Here's how the part is built. I have some questions about the finished solid (model axes, mm). Face numbers are marked on the shaded views. A direction names the side the tool comes from. Coordinates: 2 decimals unless noted, no trailing zeros. Loops run counter-clockwise (first coordinate to the right, second up) from the corner with the lowest first, then second, coordinate; pieces in that order, holes last. Notation, with made-up numbers: (2, 13) -> (45, 13) arc R19 cw to (45, 35) -> close; hole circle Ø10 at (61.25, 12). An arc over 180 degrees is marked (long way). Answer as a JSON object with one key per item and string values. Group by question number.
1) I want a section at A-A (y = 0). Write out the boundary of the cut face in (x, z) (3 decimals), then the cut area to 3 significant figures.
2) I need wall thicknesses on probe 1 along Y at (x, z) = (0, 4.6) (3 decimals); probe 2 along Y at (x, z) = (0, 0.45); probe 3 along X at (y, z) = (0, 1). Which ranges of each line are inside material? Lowest first, please. Write a range as [from, to].
3) Which directions (+Z, -Z, +X, -X, +Y, -Y) give clear straight access to the entire face, cutting with the end or side of a thin tool? Please do the marked faces 1, 2 and 3.
4) I'm going to push flat-ended pins straight in: pin 1 (2 mm diameter, centred on x = -3.5, z = 5, fed in from +Y); pin 2 (2 mm diameter, centred on x = 2.5, z = 5, fed in from +Y); pin 3 (5.5 mm diameter, centred on x = 0, y = 0, fed in from +Z). Where does each tip first touch, or does it pass through?
5) I want a section at C-C (z = 1.3). Write out the boundary of the cut face in (x, y).
6) If we mould it in two halves opening along X, with no side actions, what happens to the marked faces 4, 5 and 6? For each: +X half, -X half, draft (parallel to the pull), parting line (faces both ways), or undercut.
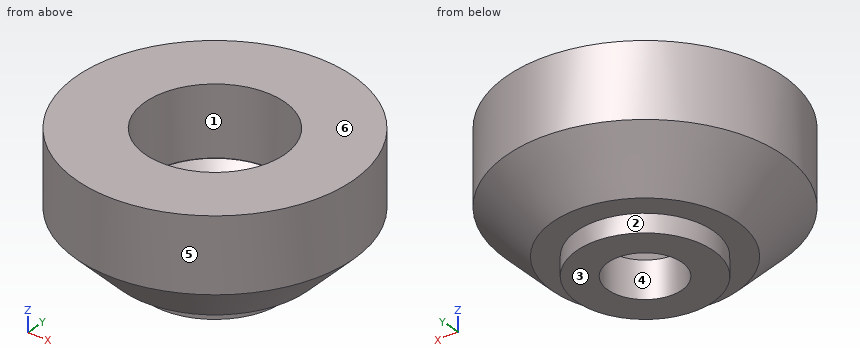
Autodesk Inventor part; units mm, degrees
ref_plane "YZ Plane" through (0, 0, 0) normal (1, 0, 0) x (0, 1, 0)
ref_plane "XZ Plane" through (0, 0, 0) normal (0, 1, 0) x (-1, 0, 0)
ref_plane "XY Plane" through (0, 0, 0) normal (0, 0, 1) x (1, 0, 0)
sketch "Sketch1" plane through (0, 0, 0) normal (0, 0, 1) x (1, 0, 0)
  circle A0 centre (0, 0) radius 6
  dimension "d0" = 12
extrude "Extrusion1" add sketch "Sketch1" along normal blind 3.5
sketch "Sketch2" plane through (0, 0, 3.5) normal (0, 0, 1) x (1, 0, 0)
  circle A0 centre (0, 0) radius 1.55
  dimension "d3" = 3.1
extrude "Extrusion2" cut sketch "Sketch2" against normal through all
sketch "Sketch3" plane through (0, 0, 0) normal (0, 0, -1) x (-1, 0, 0)
  circle A0 centre (0, 0) radius 2.96
  circle A1 centre (0, 0) radius 7.5
  dimension "d6" = 5.92
  dimension "d16" = 15
extrude "Extrusion3" cut sketch "Sketch3" against normal blind 0.8
sketch "Sketch4" plane through (0, 0, 3.5) normal (0, 0, 1) x (1, 0, 0)
  circle A0 centre (0, 0) radius 2.5
  dimension "d9" = 5
extrude "Extrusion4" cut sketch "Sketch4" against normal blind 1.5
sketch "Sketch5" plane through (0, 0, 3.5) normal (0, 0, 1) x (1, 0, 0)
  circle A0 centre (0, 0) radius 6
  circle A1 centre (0, 0) radius 2.5
  circle A2 centre (0, 0) radius 3.025
  circle A3 centre (0, 0) radius 6
  dimension "d12" = 6.05
  dimension "d15" = 0
extrude "Extrusion5" add sketch "Sketch5" along normal blind 2.5 contours A0
chamfer "Chamfer1" distance 2 angle 45 1 edges at (-6, 0, 0.8)
sketch "Sketch6" plane through (0, 0, 3.5) normal (0, 0, 1) x (1, 0, 0)
  circle A0 centre (0, 0) radius 3.025
  circle A1 centre (0, 0) radius 2.5
extrude "Extrusion6" cut sketch "Sketch6" against normal up to surface (1.5 mm away)
sketch "Sketch7" plane through (0, 0, 2) normal (0, 0, 1) x (1, 0, 0)
  circle A0 centre (0, 0) radius 3.025
  circle A1 centre (0, 0) radius 1.55
extrude "Extrusion7" add sketch "Sketch7" along normal blind 1
sketch "Sketch8" plane through (0, 0, 3) normal (0, 0, 1) x (1, 0, 0)
  point P0 (0, 0)
hole "Hole1" at (0, 0, 3) direction (0, 0, -1) diameter 3.2 end through all countersink diameter 6 countersink angle 90
properties part number "motor_and_magnet_holder"
Determined:
{
 "1": {"outline": "(-6, 2.8) -> (-4, 0.8) -> (-2.96, 0.8) -> (-2.96, 0) -> (-1.6, 0) -> (-1.6, 1.6) -> (-3, 3) -> (-3.025, 3) -> (-3.025, 6) -> (-6, 6) -> close; (1.6, 0) -> (2.96, 0) -> (2.96, 0.8) -> (4, 0.8) -> (6, 2.8) -> (6, 6) -> (3.025, 6) -> (3.025, 3) -> (3, 3) -> (1.6, 1.6) -> close", "area": "33.4 mm^2"},
 "2": {"probe 1": "[-6, -3.025], [3.025, 6]", "probe 2": "[-2.96, -1.6], [1.6, 2.96]", "probe 3": "[-4.2, -1.6], [1.6, 4.2]"},
 "3": {"face 1": "+Z", "face 2": "-Z", "face 3": "-Z, +X, -X, +Y, -Y"},
 "4": {"pin 1": "y = 5.45", "pin 2": "y = 5.81", "pin 3": "z = 2.75"},
 "5": {"outline": "circle Ø9 at (0, 0); hole circle Ø3.2 at (0, 0)"},
 "6": {"face 4": "undercut", "face 5": "parting line", "face 6": "draft"}
}
